from build123d import *

# Parameters (mm, degrees)
BOSS_EXTRUDE1_DEPTH  = 4
SKETCH2_R            = 2.5
BOSS_EXTRUDE2_DEPTH  = 3
SKETCH5_R            = 4.5
SKETCH3_R            = 8.5
SKETCH6_R            = 3
CUT_EXTRUDE1_DEPTH   = 24.456289064
SKETCH7_W            = 90
SKETCH7_H            = 22.544950424
BOSS_EXTRUDE3_DEPTH  = 4
BOSS_EXTRUDE4_DEPTH  = 5
CUT_EXTRUDE2_DEPTH   = 2
CUT_EXTRUDE3_START   = -2
CUT_EXTRUDE3_DEPTH   = 2
FILLET1_R            = 2
SKETCH12_W           = 13
SKETCH12_H           = 12
CUT_EXTRUDE4_DEPTH   = 2
BOSS_EXTRUDE9_REACH  = 109.642
SKETCH13_R           = 14.22
CUT_EXTRUDE5_START   = -4
SKETCH14_R           = 14.22
CUT_EXTRUDE5_DEPTH   = 4
FILLET2_R            = 50
FILLET3_R            = 50
FILLET4_R            = 2
SKETCH15_R           = 9.5
BOSS_EXTRUDE10_DEPTH = 2.9
BOSS_EXTRUDE10_TAPER = 30
SKETCH16_R           = 3.5
CUT_EXTRUDE6_DEPTH   = 131.409814092
SKETCH17_R           = 1.5
CUT_EXTRUDE7_DEPTH   = 131.481069935
CUT_EXTRUDE8_DEPTH   = 3
CUT_EXTRUDE9_DEPTH   = 3


with BuildPart() as part:
    # Sketch1 → Boss-Extrude1 (new body)
    with BuildSketch(Plane.XY):
        with BuildLine():
            Line((1.17473573, 8.923003752), (-16.671271775, 11.272475212))
            ThreePointArc((-16.671271775, 11.272475212), (-19.953165144, 0), (-16.671271775, -11.272475212))
            Line((-16.671271775, -11.272475212), (1.17473573, -8.923003752))
            ThreePointArc((1.17473573, -8.923003752), (9, 0), (1.17473573, 8.923003752))
        make_face()
    extrude(amount=BOSS_EXTRUDE1_DEPTH)

    # Sketch2 → Boss-Extrude2 (add)
    with BuildSketch(Plane.XY.offset(4)):
        with Locations((-16, 0)):
            Circle(SKETCH2_R)
    extrude(amount=BOSS_EXTRUDE2_DEPTH)

    # Sketch5 → Loft1 section 0
    with BuildSketch(Plane.XY.offset(5)):
        Circle(SKETCH5_R)
    # Sketch3 → Loft1 section 1
    with BuildSketch(Plane.XY.offset(4)):
        Circle(SKETCH3_R)
    loft()

    # Sketch6 → Cut-Extrude1 (cut, through all)
    with BuildSketch(Plane.XY.offset(5)):
        Circle(SKETCH6_R)
    extrude(amount=-CUT_EXTRUDE1_DEPTH, mode=Mode.SUBTRACT)

    # Sketch7 → Boss-Extrude3 (add)
    with BuildSketch(Plane.XY.offset(4)):
        with Locations((-61.671271775, 0)):
            Rectangle(SKETCH7_W, SKETCH7_H)
    extrude(amount=-BOSS_EXTRUDE3_DEPTH)

    # Sketch8 → Boss-Extrude4 (add)
    with BuildSketch(Plane.XY.offset(4)):
        with BuildLine():
            Line((-106.671271775, 11.272475212), (-21.671271775, 11.272475212))
            ThreePointArc((-21.671271775, 11.272475212), (-24.316626975, 0), (-21.671271775, -11.272475212))
            Line((-21.671271775, -11.272475212), (-106.671271775, -11.272475212))
            Line((-106.671271775, -11.272475212), (-106.671271775, 11.272475212))
        make_face()
    extrude(amount=BOSS_EXTRUDE4_DEPTH)

    # Sketch9 → Cut-Extrude2 (cut)
    with BuildSketch(Plane(origin=(0, 0, 0), x_dir=(-1, 0, 0), z_dir=(0, 0, -1))):
        with BuildLine():
            Line((23.091271775, 5), (8.091271775, 3.025212536))
            ThreePointArc((8.091271775, 3.025212536), (8.583093751, 0), (8.091271775, -3.025212536))
            Line((8.091271775, -3.025212536), (23.091271775, -5))
            Line((23.091271775, -5), (106.671271775, -5))
            Line((106.671271775, -5), (106.671271775, 5))
            Line((106.671271775, 5), (23.091271775, 5))
        make_face()
    extrude(amount=-CUT_EXTRUDE2_DEPTH, mode=Mode.SUBTRACT)

    # Sketch11 → Cut-Extrude3 (cut)
    with BuildSketch(Plane.XY.offset(9).offset(CUT_EXTRUDE3_START)):
        with BuildLine():
            Line((-106.671271775, 5), (-23.818438503, 5))
            ThreePointArc((-23.818438503, 5), (-24.316626975, 0), (-23.818438503, -5))
            Line((-23.818438503, -5), (-106.671271775, -5))
            Line((-106.671271775, -5), (-106.671271775, 5))
        make_face()
    extrude(amount=CUT_EXTRUDE3_DEPTH, mode=Mode.SUBTRACT)

    # Fillet1
    fillet1_edges = [part.edges().sort_by_distance(p)[0] for p in [
        (-65.244855139, -5, 7),
        (-65.244855139, 5, 7),
    ]]
    fillet(fillet1_edges, radius=FILLET1_R - 0.0001)  # a hair under: the kernel refuses the full size

    # Sketch12 → Cut-Extrude4 (cut)
    with BuildSketch(Plane(origin=(0, 0, 0), x_dir=(-1, 0, 0), z_dir=(0, 0, -1))):
        with Locations((100.171271775, 0)):
            Rectangle(SKETCH12_W, SKETCH12_H)
    extrude(amount=-CUT_EXTRUDE4_DEPTH, mode=Mode.SUBTRACT)

    # Boss-Extrude9: up to this face of the body (flat: up to its plane)
    boss_extrude9_end = Plane(part.part.faces().sort_by_distance((-64.78254731, 8.149583263, 9))[0])
    # Sketch13 → Boss-Extrude9 (add, up to the picked face)
    with BuildSketch(Plane(origin=(0, 0, 0), x_dir=(-1, 0, 0), z_dir=(0, 0, -1)), mode=Mode.PRIVATE) as boss_extrude9_sk1:
        with Locations((115.171271775, 0)):
            Circle(SKETCH13_R)
    boss_extrude9_tool1 = split(extrude(boss_extrude9_sk1.sketch, amount=-BOSS_EXTRUDE9_REACH, mode=Mode.PRIVATE), bisect_by=boss_extrude9_end, keep=Keep.BOTH, mode=Mode.PRIVATE)
    add(boss_extrude9_tool1.solids().sort_by(Axis((-115.171272, 0, 0), (0, 0, 1)))[0])

    # Sketch14 → Cut-Extrude5 (cut)
    with BuildSketch(Plane.XY.offset(9).offset(CUT_EXTRUDE5_START)):
        with Locations((-115.171271775, 0)):
            Circle(SKETCH14_R)
    extrude(amount=CUT_EXTRUDE5_DEPTH, mode=Mode.SUBTRACT)

    # Fillet2
    fillet2_edges = [part.edges().sort_by_distance(p)[0] for p in [
        (-106.502955757, -11.272475212, 2.5),
    ]]
    fillet(fillet2_edges, radius=FILLET2_R)

    # Fillet3
    fillet3_edges = [part.edges().sort_by_distance(p)[0] for p in [
        (-106.502955757, 11.272475212, 2.5),
    ]]
    fillet(fillet3_edges, radius=FILLET3_R)

    # Fillet4
    fillet4_edges = [part.edges().sort_by_distance(p)[0] for p in [
        (-106.502955757, 11.272475212, 7),
        (-106.502955757, -11.272475212, 7),
    ]]
    fillet(fillet4_edges, radius=FILLET4_R)

    # Sketch15 → Boss-Extrude10 (add)
    with BuildSketch(Plane.XY.offset(5)):
        with Locations((-115.171271775, 0)):
            Circle(SKETCH15_R)
    extrude(amount=BOSS_EXTRUDE10_DEPTH, taper=BOSS_EXTRUDE10_TAPER)

    # Sketch16 → Cut-Extrude6 (cut, through all)
    with BuildSketch(Plane.XY.offset(7.9)):
        with Locations((-115.171271775, 0)):
            Circle(SKETCH16_R)
    extrude(amount=-CUT_EXTRUDE6_DEPTH, mode=Mode.SUBTRACT)

    # Sketch17 → Cut-Extrude7 (cut, through all)
    with BuildSketch(Plane.XY.offset(9)):
        with Locations((-98.64, 8.37)):
            Circle(SKETCH17_R)
        with Locations((-98.64, -8.37)):
            Circle(SKETCH17_R)
        with Locations((-28.64, -8.37)):
            Circle(SKETCH17_R)
        with Locations((-28.64, 8.37)):
            Circle(SKETCH17_R)
    extrude(amount=-CUT_EXTRUDE7_DEPTH, mode=Mode.SUBTRACT)

    # Sketch18 → Cut-Extrude8 (cut)
    with BuildSketch(Plane(origin=(0, 0, 0), x_dir=(-1, 0, 0), z_dir=(0, 0, -1))):
        with BuildLine():
            Line((116.629965164, -7.68), (117.419965164, -4.48))
            ThreePointArc((117.419965164, -4.48), (117.675667138, -3.719084235), (118.209965164, -3.12))
            ThreePointArc((118.209965164, -3.12), (118.224204792, -3.109259088), (118.238318816, -3.098353652))
            ThreePointArc((118.238318816, -3.098353652), (118.249224252, -3.084239628), (118.259965164, -3.07))
            ThreePointArc((118.259965164, -3.07), (118.859049399, -2.535701974), (119.619965164, -2.28))
            Line((119.619965164, -2.28), (122.819965164, -1.49))
            ThreePointArc((122.819965164, -1.49), (123.762740802, -0.995512646), (124.139965164, 0))
            ThreePointArc((124.139965164, 0), (123.762740802, 0.995512646), (122.819965164, 1.49))
            Line((122.819965164, 1.49), (119.619965164, 2.28))
            ThreePointArc((119.619965164, 2.28), (118.859049399, 2.535701974), (118.259965164, 3.07))
            ThreePointArc((118.259965164, 3.07), (118.249224252, 3.084239628), (118.238318816, 3.098353652))
            ThreePointArc((118.238318816, 3.098353652), (118.224204792, 3.109259088), (118.209965164, 3.12))
            ThreePointArc((118.209965164, 3.12), (117.675667138, 3.719084235), (117.419965164, 4.48))
            Line((117.419965164, 4.48), (116.629965164, 7.68))
            ThreePointArc((116.629965164, 7.68), (116.135477809, 8.622775638), (115.139965164, 9))
            ThreePointArc((115.139965164, 9), (114.144452518, 8.622775638), (113.649965164, 7.68))
            Line((113.649965164, 7.68), (112.859965164, 4.48))
            ThreePointArc((112.859965164, 4.48), (112.60426319, 3.719084235), (112.069965164, 3.12))
            ThreePointArc((112.069965164, 3.12), (112.055725536, 3.109259088), (112.041611512, 3.098353652))
            ThreePointArc((112.041611512, 3.098353652), (112.030706076, 3.084239628), (112.019965164, 3.07))
            ThreePointArc((112.019965164, 3.07), (111.420880929, 2.535701974), (110.659965164, 2.28))
            Line((110.659965164, 2.28), (107.459965164, 1.49))
            ThreePointArc((107.459965164, 1.49), (106.517189526, 0.995512646), (106.139965164, 0))
            ThreePointArc((106.139965164, 0), (106.517189526, -0.995512646), (107.459965164, -1.49))
            Line((107.459965164, -1.49), (110.659965164, -2.28))
            ThreePointArc((110.659965164, -2.28), (111.420880929, -2.535701974), (112.019965164, -3.07))
            ThreePointArc((112.019965164, -3.07), (112.030706076, -3.084239628), (112.041611512, -3.098353652))
            ThreePointArc((112.041611512, -3.098353652), (112.055725536, -3.109259088), (112.069965164, -3.12))
            ThreePointArc((112.069965164, -3.12), (112.60426319, -3.719084235), (112.859965164, -4.48))
            Line((112.859965164, -4.48), (113.649965164, -7.68))
            ThreePointArc((113.649965164, -7.68), (114.144452518, -8.622775638), (115.139965164, -9))
            ThreePointArc((115.139965164, -9), (116.135477809, -8.622775638), (116.629965164, -7.68))
        make_face()
    extrude(amount=-CUT_EXTRUDE8_DEPTH, mode=Mode.SUBTRACT)

    # Sketch19 → Cut-Extrude9 (cut)
    with BuildSketch(Plane(origin=(0, 0, 0), x_dir=(-1, 0, 0), z_dir=(0, 0, -1))):
        with BuildLine():
            Line((-1.2, 6.33), (-1.8, 4.16))
            ThreePointArc((-1.8, 4.16), (-2.089343599, 3.728660349), (-2.48, 3.386372183))
            ThreePointArc((-2.48, 3.386372183), (-2.740944688, 3.196252087), (-2.985706385, 2.985706385))
            ThreePointArc((-2.985706385, 2.985706385), (-3.196252087, 2.740944688), (-3.386372183, 2.48))
            ThreePointArc((-3.386372183, 2.48), (-3.728660349, 2.089343599), (-4.16, 1.8))
            Line((-4.16, 1.8), (-6.33, 1.2))
            ThreePointArc((-6.33, 1.2), (-6.992020752, 0.754882576), (-7.25, 0))
            ThreePointArc((-7.25, 0), (-6.992020752, -0.754882576), (-6.33, -1.2))
            Line((-6.33, -1.2), (-4.16, -1.8))
            ThreePointArc((-4.16, -1.8), (-3.728660349, -2.089343599), (-3.386372183, -2.48))
            ThreePointArc((-3.386372183, -2.48), (-3.196252087, -2.740944688), (-2.985706385, -2.985706385))
            ThreePointArc((-2.985706385, -2.985706385), (-2.740944688, -3.196252087), (-2.48, -3.386372183))
            ThreePointArc((-2.48, -3.386372183), (-2.089343599, -3.728660349), (-1.8, -4.16))
            Line((-1.8, -4.16), (-1.2, -6.33))
            ThreePointArc((-1.2, -6.33), (-0.754882576, -6.992020752), (0, -7.25))
            ThreePointArc((0, -7.25), (0.754882576, -6.992020752), (1.2, -6.33))
            Line((1.2, -6.33), (1.8, -4.16))
            ThreePointArc((1.8, -4.16), (2.089343599, -3.728660349), (2.48, -3.386372183))
            ThreePointArc((2.48, -3.386372183), (2.740944688, -3.196252087), (2.985706385, -2.985706385))
            ThreePointArc((2.985706385, -2.985706385), (3.196252087, -2.740944688), (3.386372183, -2.48))
            ThreePointArc((3.386372183, -2.48), (3.728660349, -2.089343599), (4.16, -1.8))
            Line((4.16, -1.8), (6.33, -1.2))
            ThreePointArc((6.33, -1.2), (6.992020752, -0.754882576), (7.25, 0))
            ThreePointArc((7.25, 0), (6.992020752, 0.754882576), (6.33, 1.2))
            Line((6.33, 1.2), (4.16, 1.8))
            ThreePointArc((4.16, 1.8), (3.728660349, 2.089343599), (3.386372183, 2.48))
            ThreePointArc((3.386372183, 2.48), (3.196252087, 2.740944688), (2.985706385, 2.985706385))
            ThreePointArc((2.985706385, 2.985706385), (2.740944688, 3.196252087), (2.48, 3.386372183))
            ThreePointArc((2.48, 3.386372183), (2.089343599, 3.728660349), (1.8, 4.16))
            Line((1.8, 4.16), (1.2, 6.33))
            ThreePointArc((1.2, 6.33), (0.754882576, 6.992020752), (0, 7.25))
            ThreePointArc((0, 7.25), (-0.754882576, 6.992020752), (-1.2, 6.33))
        make_face()
    extrude(amount=-CUT_EXTRUDE9_DEPTH, mode=Mode.SUBTRACT)


solid = part.part
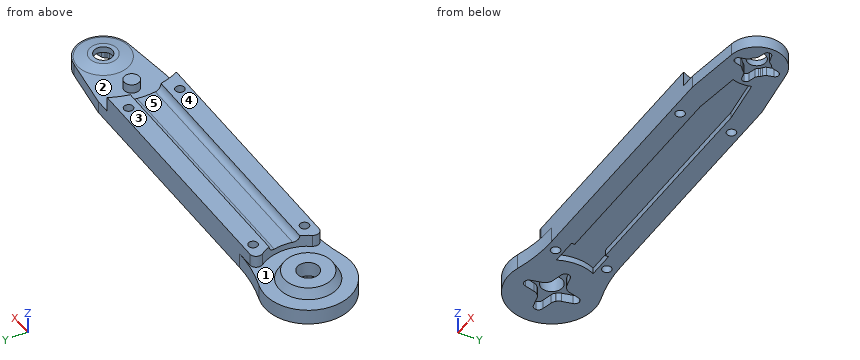
Check sheet for the modelled part. Datum: model origin and axes. Units: mm. Face numbers are marked on the shaded views. A direction names the side the tool comes from. Give positions to 0.01 mm unless a question says otherwise; leave off trailing zeros. Answer as CSV lines item,"result". Start each with the question number.
Item 1: Gauge pin test, flat ends, axial feed: P1, Ø6.5, axis at x = -77.5, y = 0.5, coming from the +Z side; P2, Ø1, axis at x = -98, z = 1, coming from the -Y side; P3, Ø1, axis at x = -99, z = 1.5, coming from the +Y side; P4, Ø11, axis at x = -115.17, y = 0, coming from the -Z side. Record the tip position at first contact, or that the pin passes through.
Item 2: Cross-section at B-B on x = -98.64. State how many separate pieces and enclosed holes the cut face has, plus the area to 3 significant figures.
Item 3: Mould release check, pull along X, two halves, no side actions. Record for the marked faces 1, 2 and 3: +X half, -X half, draft (parallel to the pull), parting line (faces both ways), or undercut.
Item 4: Tool access check on the marked faces 4 and 5. Record the directions out of +Z, -Z, +X, -X, +Y, -Y that give a thin tool (end or side, any length) a straight path to the whole face; none if there is none.
Item 5: Thickness scan on line 1 (Y direction, x = -3, z = 1.5); line 2 (Y direction, x = -28.64, z = 6.5); line 3 (Y direction, x = -98, z = 2.25). Record the ranges inside material, lowest first. Write a range as [from, to].
Established:
1,P1,"stops at z = 7.15"
1,P2,"stops at y = -11.34"
1,P3,"stops at y = 11.4"
1,P4,"stops at z = 0"
2,separate pieces,"3"
2,enclosed holes,"0"
2,area,"107 mm^2"
3,face 1,"undercut"
3,face 2,"undercut"
3,face 3,"draft"
4,face 4,"+Z, +X, -X, +Y, -Y"
4,face 5,"+Z, +X"
5,line 1,"y = [-9.47, -2.97], [2.97, 9.47]"
5,line 2,"y = [-11.27, -9.87], [-6.87, 6.87], [9.87, 11.27]"
5,line 3,"y = [-11.31, -9.73], [-7.01, 7.01], [9.73, 11.31]"
